Autodesk Inventor part; units mm, degrees
ref_plane "YZ Plane" through (0, 0, 0) normal (1, 0, 0) x (0, 1, 0)
ref_plane "XZ Plane" through (0, 0, 0) normal (0, 1, 0) x (-1, 0, 0)
ref_plane "XY Plane" through (0, 0, 0) normal (0, 0, 1) x (1, 0, 0)
sketch "Sketch1" plane through (0, 0, 0) normal (0, 0, 1) x (1, 0, 0)
  circle A0 centre (0, 0) radius 25.6
  circle A1 centre (0, 0) radius 57.15
  circle A2 centre (0, 44.45) radius 3.3734
  circle A3 centre (-38.4948, 22.225) radius 3.3734
  circle A4 centre (-38.4948, -22.225) radius 3.3734
  circle A5 centre (0, -44.45) radius 3.3734
  circle A6 centre (38.4948, -22.225) radius 3.3734
  circle A7 centre (38.4948, 22.225) radius 3.3734
  dimension "d0" = 51.2
  dimension "d1" = 44.45
  dimension "d2" = 6.7469
  dimension "d3" = 114.3
  dimension "d6" = 360
extrude "Extrusion1" add sketch "Sketch1" along normal blind 6.35
sketch "Sketch2" plane through (0, 0, 6.35) normal (0, 0, 1) x (1, 0, 0)
  circle A0 centre (0, 0) radius 31.95
  circle A1 centre (0, 0) radius 25.6
  dimension "d10" = 6.35
extrude "Extrusion2" add sketch "Sketch2" along normal blind 12.7
properties part number "IndexerWheelBushing"
Could you check a few things on this model? Use its own coordinates, in mm. A direction names the side the tool comes from. Round coordinates to 2 decimals unless told otherwise and drop trailing zeros. Loops run counter-clockwise (first coordinate to the right, second up) from the corner with the lowest first, then second, coordinate; pieces in that order, holes last. Notation, with made-up numbers: (39, 16.25) -> (80, 16.25) arc R13 cw to (80, 39.25) -> close; hole circle Ø8 at (-13.5, 24). An arc over 180 degrees is marked (long way). Use CSV: the item, a comma, the result in double quotes.
(1) Suppose I cut it at A-A on y = 0. Write out the boundary of the cut face in (x, z).
Return value:
outline,"(-57.15, 0) -> (-25.6, 0) -> (-25.6, 19.05) -> (-31.95, 19.05) -> (-31.95, 6.35) -> (-57.15, 6.35) -> close; (25.6, 0) -> (57.15, 0) -> (57.15, 6.35) -> (31.95, 6.35) -> (31.95, 19.05) -> (25.6, 19.05) -> close"
(2) Suppose I cut it at B-B on x = 0. Write out the boundary of the cut face in (y, z), plus the area to 3 significant figures.
Return value:
outline,"(-57.15, 0) -> (-47.82, 0) -> (-47.82, 6.35) -> (-57.15, 6.35) -> close; (-41.08, 0) -> (-25.6, 0) -> (-25.6, 19.05) -> (-31.95, 19.05) -> (-31.95, 6.35) -> (-41.08, 6.35) -> close; (25.6, 0) -> (41.08, 0) -> (41.08, 6.35) -> (31.95, 6.35) -> (31.95, 19.05) -> (25.6, 19.05) -> close; (47.82, 0) -> (57.15, 0) -> (57.15, 6.35) -> (47.82, 6.35) -> close"
area,"476 mm²"
(3) Will these pins go through, and if not, where does the flat tip stop? pin 1 Ø3 at (y, z) = (-20.5, 3) entering from +X; pin 2 Ø1 at (x, z) = (37.5, 8) entering from +Y; pin 3 Ø11 at (x, y) = (0, -44.45) entering from +Z; pin 4 Ø2 at (x, z) = (-34.5, 3.5) entering from +Y.
Return value:
pin 1,"stops at x = 53.9"
pin 2,"passes through"
pin 3,"stops at z = 6.35"
pin 4,"stops at y = 46.3"
(4) Suppose I cut it at C-C on z = 8.5. Write out the boundary of the cut face in (x, y).
Return value:
outline,"circle Ø63.9 at (0, 0); hole circle Ø51.2 at (0, 0)"
(5) If we mould it in two halves opening along Y, with no side actions, what happens to faces 3 (the cylindrical face through (40.31, -25.07, 3.13)), 4 (the cylindrical face through (-57.095, -2.513, 3.131)), 5 (the flat face through (25, -25, 6.35))? For each: +Y half, -Y half, draft (parallel to the pull), parting line (faces both ways), or undercut.
Return value:
face 3,"undercut"
face 4,"parting line"
face 5,"draft"
(6) For faces 1 (the cylindrical face through (-0.4, -47.8, 3.1)), 2 (the cylindrical face through (-6.93, 31.19, 12.61)), which set-ups out of +Z, -Z, +X, -X, +Y, -Y let a thin tool reach every point of the face, with its end or its side?
Return value:
face 1,"+Z, -Z"
face 2,"+Z"
(7) Suppose I cut it at D-D on y = 46. Write out the boundary of the cut face in (x, z), plus the area to 3 significant figures.
Return value:
outline,"(-33.91, 0) -> (-3, 0) -> (-3, 6.35) -> (-33.91, 6.35) -> close; (3, 0) -> (33.91, 0) -> (33.91, 6.35) -> (3, 6.35) -> close"
area,"393 mm²"
(8) If I drill on probe 1 along Y at (x, z) = (0, 2.5); probe 2 along Z at (x, y) = (51, 1.5); probe 3 along X at (y, z) = (-20.5, 16), over which ranges is the centre line in solid material (lowest first)? Write a range as [from, to].
Return value:
probe 1,"y = [-57.15, -47.82], [-41.08, -25.6], [25.6, 41.08], [47.82, 57.15]"
probe 2,"z = [0, 6.35]"
probe 3,"x = [-24.51, -15.33], [15.33, 24.51]"
